For this review, use the dimensioned drawing (mm, ordinates from the lowest corner) and the shaded views. A direction names the side the tool comes from. Give positions to 0.01 mm unless a question says otherwise; leave off trailing zeros. Loops run counter-clockwise (first coordinate to the right, second up) from the corner with the lowest first, then second, coordinate; pieces in that order, holes last. Notation, with made-up numbers: M 47,47 L 57,47 A16 cw 57,56 Z; hole C 80,-8.75 d7. An arc over 180 degrees is marked long. Use CSV: the item, a comma, the result in double quotes. Start each with the question number.
1. Take a section at B-B, the plane z = 24. Write out the cut boundary in (x, y), and give its area (3 significant figures).
2. To check wall thickness, follow line 1 (X direction, y = 22, z = 22); line 2 (Y direction, x = 54, z = 5.5); line 3 (Z direction, x = 67.5, y = 27). State the ranges of each line that lie inside material, in increasing order. Write a range as [from, to].
3. Take a section at C-C, the plane y = 23. Write out the cut boundary in (x, z) (1 decimal), and give its area (4 significant figures).
4. Insertion check: P1, Ø6, axis at x = 33.5, y = 17, coming from the +Z side; P2, Ø1.5, axis at y = 26.5, z = 39, coming from the +X side; P3, Ø10, axis at y = 25.5, z = 49.5, coming from the +X side. Each pin has a flat end and moves straight along its axis. Give the tip position at first contact, or say it passes through.
5. The part is to be moulded in two halves that separate along Z. For the marked faces 6, 7 and 8, say which applies: pulls with the +Z half, pulls with the -Z half, needs draft (parallel to the pull), parting line crosses it, or undercut.
6. Take a section at A-A, the plane x = 21.5. Write out the cut boundary in (y, z).
7. Take a section at D-D, the plane z = 50. Write out the cut boundary in (x, y), and give its area (3 significant figures).
8. Tool access review of the marked faces 1, 2, 3, 4 and 5: name each direction out of +Z, -Z, +X, -X, +Y, -Y from which nothing blocks a thin tool from reaching the whole face with its end or side.
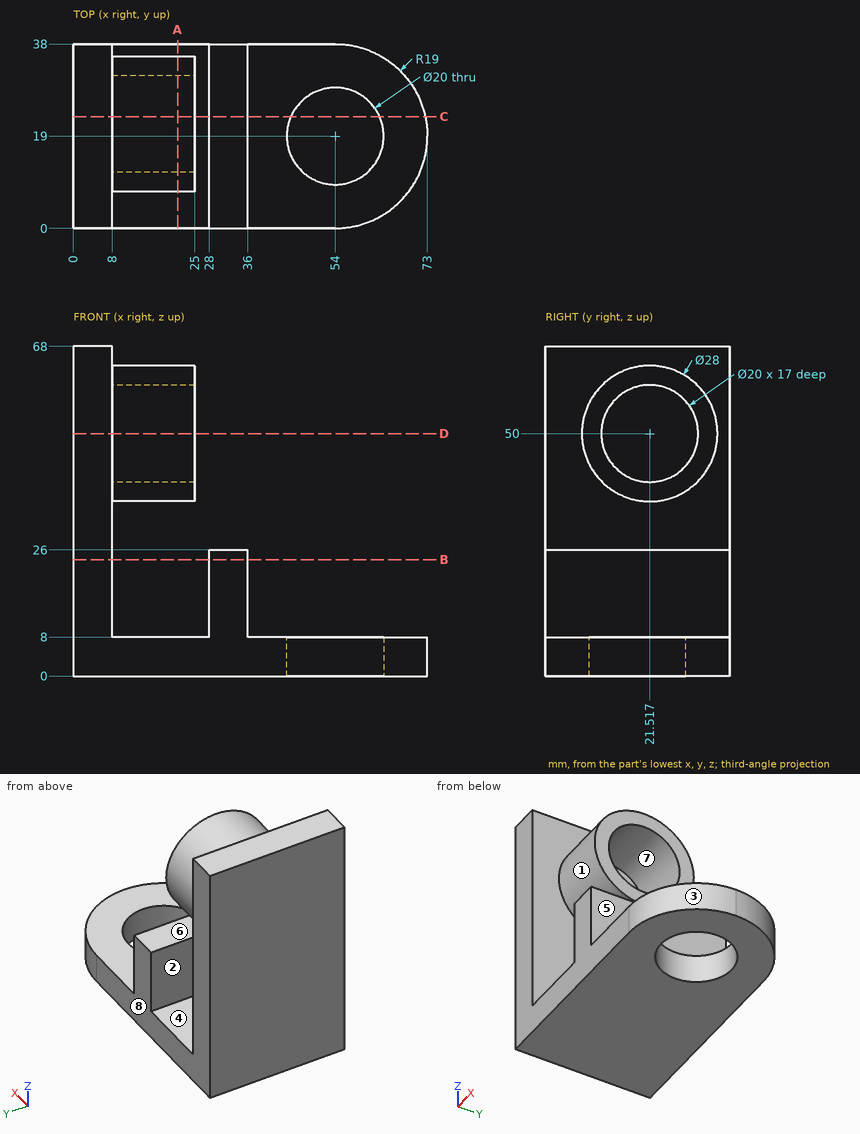
Result set:
1,outline,"M 0,0 L 8,0 L 8,38 L 0,38 Z; M 28,0 L 36,0 L 36,38 L 28,38 Z"
1,area,"608 mm2"
2,line 1,"[0, 8], [28, 36]"
2,line 2,"[0, 9], [29, 38]"
2,line 3,"[0, 8]"
3,outline,"M 0,0 L 44.8,0 L 44.8,8 L 36,8 L 36,26 L 28,26 L 28,8 L 8,8 L 8,36.1 L 25,36.1 L 25,40.1 L 8,40.1 L 8,59.9 L 25,59.9 L 25,63.9 L 8,63.9 L 8,68 L 0,68 Z; M 63.2,0 L 72.6,0 L 72.6,8 L 63.2,8 Z"
3,area,"1,195 mm2"
4,P1,"z = 26"
4,P2,"x = 25"
4,P3,"x = 8"
5,face 6,"pulls with the +Z half"
5,face 7,"undercut"
5,face 8,"needs draft"
6,outline,"M 0,0 L 38,0 L 38,8 L 0,8 Z; C 21.52,50 d28; hole C 21.52,50 d20"
7,outline,"M 0,0 L 8,0 L 8,7.52 L 25,7.52 L 25,11.52 L 8,11.52 L 8,31.52 L 25,31.52 L 25,35.52 L 8,35.52 L 8,38 L 0,38 Z"
7,area,"440 mm2"
8,face 1,"+X"
8,face 2,"+Z, +Y, -Y"
8,face 3,"+Z, -Z, +X, -Y"
8,face 4,"+Y, -Y"
8,face 5,"+Z, +X, +Y, -Y"
